Source: CAD feature listing. Evaluate the final solid. Frame: model axes, mm. Face numbers are marked on the shaded views. A direction names the side the tool comes from. Give positions to 0.01 mm unless a question says otherwise; leave off trailing zeros. Loops run counter-clockwise (first coordinate to the right, second up) from the corner with the lowest first, then second, coordinate; pieces in that order, holes last. Notation, with made-up numbers: (-31.75, 30) -> (12.25, 30) arc R21 cw to (12.25, 48) -> close; hole circle Ø5 at (47, -33). An arc over 180 degrees is marked (long way). Return JSON: item names as keys, results as strings. Group by question number.
(1) Pin query (flat end, axial travel): pin 1 (2.5 mm diameter, centred on x = 6, z = 0, fed in from +Y). Return the tip coordinate at first contact, or that it passes through.
(2) Draft query along X for the marked faces 3, 4, 5 and 6. Return one class per face: released by +X, released by -X, zero draft, split by the parting line, or undercut.
(3) Cut plane C-C on x = 0. Return loops of the section in (y, z), then the cut area to 3 significant figures.
(4) Cut plane B-B on y = 1.2. Return loops of the section in (x, z), then the cut area to 3 significant figures.
(5) Cut plane A-A on z = 0. Return loops of the section in (x, y).
(6) Ray query, line 1 (X direction, y = 1.15, z = 0); line 2 (Y direction, x = 10.75, z = -2); line 3 (Z direction, x = 6, y = 1.45). Return the intervals inside material, ascending. Write a range as from..to.
(7) Access query for the marked faces 1 and 2. Directions: +Z, -Z, +X, -X, +Y, -Y. A direction counts if a zero-diameter tool reaches every point of the face in a straight line with its end or side. Return the directions, or none.
(8) Cut plane D-D on x = 11. Return loops of the section in (y, z).
```python
from build123d import *

# Parameters (mm, degrees)
SKETCH1_R           = 1
BOSS_EXTRUDE1_DEPTH = 2
SKETCH2_R           = 3.75
BOSS_EXTRUDE2_DEPTH = 1
SKETCH3_R           = 2.75
CUT_EXTRUDE1_DEPTH  = 1


with BuildPart() as part:
    # Sketch1 → Boss-Extrude1 (new body)
    with BuildSketch(Plane(origin=(0, 0, 0), x_dir=(1, 0, 0), z_dir=(0, 1, 0))):
        with BuildLine():
            Line((0.340909091, 3.734471983), (16.704545455, 2.24068319))
            ThreePointArc((16.704545455, 2.24068319), (18.75, 0), (16.704545455, -2.24068319))
            Line((16.704545455, -2.24068319), (0.340909091, -3.734471983))
            ThreePointArc((0.340909091, -3.734471983), (-3.75, 0), (0.340909091, 3.734471983))
        make_face()
        with Locations((6, 0)):
            Circle(SKETCH1_R, mode=Mode.SUBTRACT)
        with Locations((8.5, 0)):
            Circle(SKETCH1_R, mode=Mode.SUBTRACT)
        with Locations((11, 0)):
            Circle(SKETCH1_R, mode=Mode.SUBTRACT)
        with Locations((13.5, 0)):
            Circle(SKETCH1_R, mode=Mode.SUBTRACT)
    extrude(amount=BOSS_EXTRUDE1_DEPTH)

    # Sketch2 → Boss-Extrude2 (add)
    with BuildSketch(Plane(origin=(0, 2, 0), x_dir=(1, 0, 0), z_dir=(0, 1, 0))):
        Circle(SKETCH2_R)
    extrude(amount=BOSS_EXTRUDE2_DEPTH)

    # Sketch3 → Cut-Extrude1 (cut)
    with BuildSketch(Plane.XZ):
        Circle(SKETCH3_R)
    extrude(amount=-CUT_EXTRUDE1_DEPTH, mode=Mode.SUBTRACT)


solid = part.part
```
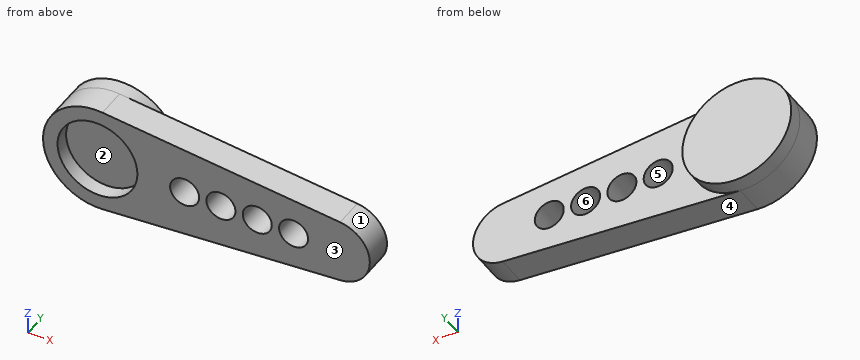
Answers:
{
 "1": {"pin 1": "y = 2"},
 "2": {"face 3": "zero draft", "face 4": "released by +X", "face 5": "undercut", "face 6": "undercut"},
 "3": {"outline": "(0, -3.75) -> (3, -3.75) -> (3, 3.75) -> (0, 3.75) -> (0, 2.75) -> (1, 2.75) -> (1, -2.75) -> (0, -2.75) -> close", "area": "17.0 mm²"},
 "4": {"outline": "(0.34, -3.73) -> (16.7, -2.24) arc R2.25 ccw to (16.7, 2.24) -> (0.34, 3.73) arc R3.75 ccw (long way) to start; hole circle Ø2 at (6, 0); hole circle Ø2 at (8.5, 0); hole circle Ø2 at (11, 0); hole circle Ø2 at (13.5, 0)", "area": "117 mm²"},
 "5": {"outline": "(-3.75, 0) -> (-2.75, 0) -> (-2.75, 1) -> (2.75, 1) -> (2.75, 0) -> (5, 0) -> (5, 2) -> (3.75, 2) -> (3.75, 3) -> (-3.75, 3) -> close; (7, 0) -> (7.5, 0) -> (7.5, 2) -> (7, 2) -> close; (9.5, 0) -> (10, 0) -> (10, 2) -> (9.5, 2) -> close; (12, 0) -> (12.5, 0) -> (12.5, 2) -> (12, 2) -> close; (14.5, 0) -> (18.75, 0) -> (18.75, 2) -> (14.5, 2) -> close"},
 "6": {"line 1": "-3.75..5, 7..7.5, 9.5..10, 12..12.5, 14.5..18.75", "line 2": "0..2", "line 3": "-3.22..-1, 1..3.22"},
 "7": {"face 1": "+X, +Y, -Y", "face 2": "-Y"},
 "8": {"outline": "(0, -2.76) -> (2, -2.76) -> (2, -1) -> (0, -1) -> close; (0, 1) -> (2, 1) -> (2, 2.76) -> (0, 2.76) -> close"}
}
